Can you work these out from the model? Positions are in its coordinate system, mm. A direction names the side the tool comes from. Round coordinates to 2 decimals unless told otherwise and drop trailing zeros. Loops run counter-clockwise (first coordinate to the right, second up) from the corner with the lowest first, then second, coordinate; pieces in that order, holes last. Notation, with made-up numbers: (84.5, 51.25) -> (89.5, 51.25) arc R20 cw to (89.5, 90.25) -> close; hole circle Ø10 at (84, -31). An arc over 180 degrees is marked (long way). Write item = value, one per line.
from build123d import *

# Parameters (mm, degrees)
F0_W      = 31.75
F0_H      = 19.05
F1_DEPTH  = 12.7
F2_W      = 50.8
F2_H      = 12.7
F3_DEPTH  = 6.35
F4_W      = 19.05
F4_H      = 5.085397
F5_DEPTH  = 6.35
F6_W      = 12.7
F6_H      = 6.35
F7_DEPTH  = 50.8
F9_R      = 3.175
F10_DEPTH = 12.7
F8_R      = 3.175
F11_DEPTH = 19.05


with BuildPart() as f1:
    # F0 (on Top) → F1 (new body)
    with BuildSketch(Plane.XY):
        with Locations((72.506752, -19.890864)):
            Rectangle(F0_W, F0_H)
    extrude(amount=F1_DEPTH)

    # F2 (on face) → F3 (join)
    with BuildSketch(Plane.XZ.offset(29.415864)):
        with Locations((82.031752, -6.35)):
            Rectangle(F2_W, F2_H)
    extrude(amount=-F3_DEPTH)

    # F4 (on face) → F5 (cut)
    with BuildSketch(Plane.XZ.offset(29.415864)):
        with Locations((97.906752, -2.542698)):
            Rectangle(F4_W, F4_H)
    extrude(amount=-F5_DEPTH, mode=Mode.SUBTRACT)

    # F6 (on face) → F7 (join)
    with BuildSketch(Plane.YZ.offset(107.431752)):
        with Locations((-29.415864, -15.875)):
            Rectangle(F6_W, F6_H)
    extrude(amount=-F7_DEPTH)

    # F9 (on face) → F10 (cut)
    with BuildSketch(Plane.XY.offset(12.7)):
        with Locations((82.031752, -16.715864)):
            Circle(F9_R)
    extrude(amount=-F10_DEPTH, mode=Mode.SUBTRACT)

    # F8 (on face) → F11 (cut)
    with BuildSketch(Plane.XZ.offset(29.415864)):
        with Locations((66.156752, 6.35)):
            Circle(F8_R)
    extrude(amount=-F11_DEPTH, mode=Mode.SUBTRACT)


solid = f1.part
1. Suppose I cut it at B-B, the plane x = 62. List the corners of the cut face in (y, z) for me.
Entries:
outline = (-35.77, -19.05) -> (-23.07, -19.05) -> (-23.07, 0) -> (-10.37, 0) -> (-10.37, 12.7) -> (-29.42, 12.7) -> (-29.42, -12.7) -> (-35.77, -12.7) -> close
2. I'm going to push flat-ended pins straight in: pin 1 (4 mm diameter, centred on x = 71, y = -17.5, fed in from -Z); pin 2 (5 mm diameter, centred on y = -18, z = 2, fed in from +X); pin 3 (1.5 mm diameter, centred on x = 73, z = -8, fed in from -Y); pin 4 (4 mm diameter, centred on x = 66.16, z = 6.35, fed in from -Y). Where does each tip first touch, or does it pass through?
Entries:
pin_1 = 0
pin_2 = 88.38
pin_3 = -29.42
pin_4 = through
3. Suppose I cut it at C-C, the plane x = 79.5. List the corners of the cut face in (y, z) for me.
Entries:
outline = (-35.77, -19.05) -> (-23.07, -19.05) -> (-23.07, 0) -> (-18.63, 0) -> (-18.63, 12.7) -> (-29.42, 12.7) -> (-29.42, -12.7) -> (-35.77, -12.7) -> close; (-14.8, 0) -> (-10.37, 0) -> (-10.37, 12.7) -> (-14.8, 12.7) -> close
4. Suppose I cut it at A-A, the plane z = 4. List the corners of the cut face in (x, y) for me (3 decimals).
Entries:
outline = (56.632, -29.416) -> (64.022, -29.416) -> (64.022, -10.366) -> (56.632, -10.366) -> close; (68.292, -29.416) -> (88.382, -29.416) -> (88.382, -10.366) -> (68.292, -10.366) -> close; hole circle Ø6.35 at (82.032, -16.716)
5. I need wall thicknesses on line 1 (Y direction, x = 87, z = 9); line 2 (Y direction, x = 98, z = -14.5); line 3 (Z direction, x = 90.5, y = -28). Which ranges of each line are inside material? Lowest first, please. Write a range as [from, to].
Entries:
line_1 = [-29.42, -10.37]
line_2 = [-35.77, -23.07]
line_3 = [-19.05, -5.09]
6. For faces 1 (the flat face through (82, -33, -12.7)), 2 (the flat face through (82, -23.066, -10)), 3 (the flat face through (88.382, -20, 6)), which set-ups out of +Z, -Z, +X, -X, +Y, -Y let a thin tool reach every point of the face, with its end or its side?
Entries:
face_1 = +Z, +X, -X, -Y
face_2 = -Z, +X, -X, +Y
face_3 = +Z, +X, +Y, -Y
7. We'd pull the mould along Y, two halves only. Please class faces 4 (the flat face through (72, -10.366, 6)), 5 (the cylindrical face through (63, -20, 6)), 6 (the flat face through (82, -35.766, -16)), 7 (the cylindrical face through (85.06, -15.76, 6.44)): released by +Y, released by -Y, zero draft, split by the parting line, or undercut.
Entries:
face_4 = released by +Y
face_5 = zero draft
face_6 = released by -Y
face_7 = undercut
8. Suppose I cut it at D-D, the plane z = -11. List the corners of the cut face in (x, y) for me, and give its area (3 significant figures).
Entries:
outline = (56.63, -29.42) -> (107.43, -29.42) -> (107.43, -23.07) -> (56.63, -23.07) -> close
area = 323 mm²
